Geometry: final body of the model. Coordinates: model frame, mm. Face numbers are marked on the shaded views. A direction names the side the tool comes from. Coordinates: 2 decimals unless noted, no trailing zeros. Order: outer loops, then holes, each group sorted by start corner. A loop starts at its lowest first (then second) coordinate and runs counter-clockwise, first axis right, second up. Notation, with made-up numbers: (82, -17.5) -> (89, -17.5) arc R26 cw to (89, 7.5) -> close; hole circle Ø2 at (-18, 83). An arc over 180 degrees is marked (long way). Answer in a Markdown table with one row per item. Add a question column.
1) Section query A-A on y = 11.25. Return the cut outline in (x, z), then the cut area to 3 significant figures.
2) Contact query for flat-ended pins moving along their axis: P1, Ø1.2, axis at x = -45.5, y = 11, coming from the +Z side; P2, Ø1, axis at x = -40, y = 8, coming from the -Z side; P3, Ø2, axis at x = -40, z = 30, coming from the -Y side. Output: stop coordinate, or through.
3) Section query C-C on y = 0. Return the cut outline in (x, z), then the cut area to 3 significant figures.
4) Section query B-B on y = -2.75. Return the cut outline in (x, z), then the cut area to 3 significant figures.
5) Pull-direction query (Z, two-part tool) for the marked faces 1, 2 and 3; classes: +Z half, -Z half, draft (parallel to the pull), parting line (faces both ways), or undercut.
6) Ray query, line 1 (Z direction, x = -39, y = -3.25); line 2 (Z direction, x = -41.5, y = -2.5); line 3 (Z direction, x = -41.5, y = 17.5). Return the intervals inside material, ascending. Write a range as from..to.
7) Set-up query: the marked faces 4, 5, 6, 7 and 8. Return all of +Z, -Z, +X, -X, +Y, -Y with unobstructed straight access to the full face (end or side cutting, diameter ignored); none if empty.
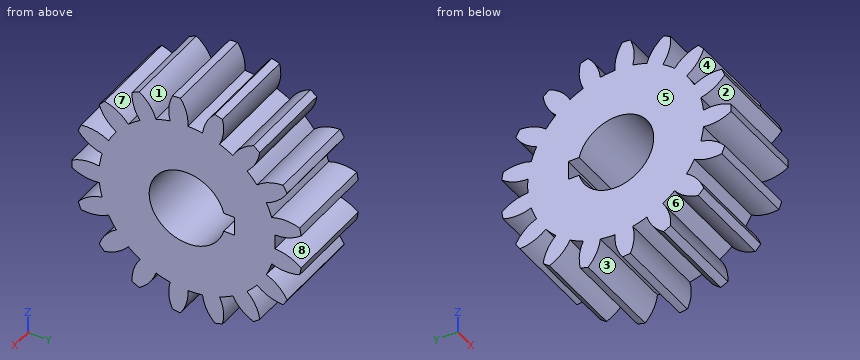
```python
from build123d import *

# Parameters (mm, degrees)
SPUR_START             = -48.138720077
SPUR_GEAR_AI_OUTLINE_R = 3.96875
SPUR_GEAR_AI_DEPTH     = 9.525
SKETCH1_W              = 2
SKETCH1_H              = 2
CUT_EXTRUDE1_DEPTH     = 39.960158194


# Read off the part's stored shape, not the designer's step: spur gear_ai
with BuildPart() as part:
    # spur gear_ai outline → spur gear_ai (new body)
    with BuildSketch(Plane.YZ.offset(SPUR_START)):
        with BuildLine():
            ThreePointArc((17.012312953, 13.95653765), (17.238554936, 14.308167954), (17.452476746, 14.667426586))
            ThreePointArc((17.452476746, 14.667426586), (16.531280061, 15.83450279), (15.268831698, 16.619929001))
            ThreePointArc((15.268831698, 16.619929001), (15.578265643, 17.328851589), (15.827189257, 18.061216004))
            ThreePointArc((15.827189257, 18.061216004), (17.289288072, 17.791147015), (18.756314792, 18.033020543))
            ThreePointArc((18.756314792, 18.033020543), (18.840255641, 18.442634067), (18.909952602, 18.854910235))
            ThreePointArc((18.909952602, 18.854910235), (17.629365722, 19.61040176), (16.168439009, 19.886740939))
            ThreePointArc((16.168439009, 19.886740939), (16.200885193, 20.659571999), (16.168439009, 21.43240306))
            ThreePointArc((16.168439009, 21.43240306), (17.629365722, 21.708742239), (18.909952602, 22.464233764))
            ThreePointArc((18.909952602, 22.464233764), (18.840255641, 22.876509932), (18.756314792, 23.286123456))
            ThreePointArc((18.756314792, 23.286123456), (17.289288072, 23.527996984), (15.827189257, 23.257927995))
            ThreePointArc((15.827189257, 23.257927995), (15.578265643, 23.99029241), (15.268831698, 24.699214998))
            ThreePointArc((15.268831698, 24.699214998), (16.531280061, 25.484641209), (17.452476746, 26.651717413))
            ThreePointArc((17.452476746, 26.651717413), (17.238554936, 27.010976045), (17.012312953, 27.362606349))
            ThreePointArc((17.012312953, 27.362606349), (15.55697648, 27.05819552), (14.291170111, 26.278192676))
            ThreePointArc((14.291170111, 26.278192676), (13.794495212, 26.871180574), (13.249864274, 27.420450766))
            ThreePointArc((13.249864274, 27.420450766), (14.143333641, 28.608887845), (14.580727415, 30.029928621))
            ThreePointArc((14.580727415, 30.029928621), (14.251472081, 30.287649847), (13.913484198, 30.533807309))
            ThreePointArc((13.913484198, 30.533807309), (12.666389228, 29.724224493), (11.767829468, 28.5396315))
            ThreePointArc((11.767829468, 28.5396315), (11.090481981, 28.913156579), (10.384209477, 29.228592392))
            ThreePointArc((10.384209477, 29.228592392), (10.788031858, 30.659535328), (10.682550269, 32.142621244))
            ThreePointArc((10.682550269, 32.142621244), (10.282429168, 32.263998384), (9.878342522, 32.371438077))
            ThreePointArc((9.878342522, 32.371438077), (9.00791614, 31.166021918), (8.597958464, 29.736824624))
            ThreePointArc((8.597958464, 29.736824624), (7.831417921, 29.840440252), (7.058889866, 29.879440332))
            ThreePointArc((7.058889866, 29.879440332), (6.918526812, 31.359632351), (6.284415731, 32.704464437))
            ThreePointArc((6.284415731, 32.704464437), (5.867467436, 32.673104837), (5.451856166, 32.627316432))
            ThreePointArc((5.451856166, 32.627316432), (5.075654279, 31.188865063), (5.209665743, 29.708084482))
            ThreePointArc((5.209665743, 29.708084482), (4.457457692, 29.527796795), (3.72300828, 29.285093965))
            ThreePointArc((3.72300828, 29.285093965), (3.057416599, 30.614626934), (1.980316242, 31.639578163))
            ThreePointArc((1.980316242, 31.639578163), (1.60285193, 31.45971711), (1.231846643, 31.266884587))
            ThreePointArc((1.231846643, 31.266884587), (1.4006774, 29.789668835), (2.060559012, 28.45729259))
            ThreePointArc((2.060559012, 28.45729259), (1.424273318, 28.017450439), (0.827094013, 27.52582306))
            ThreePointArc((0.827094013, 27.52582306), (-0.273834451, 28.525136184), (-1.648455712, 29.091781215))
            ThreePointArc((-1.648455712, 29.091781215), (-1.935457393, 28.78770994), (-2.211750379, 28.473876399))
            ThreePointArc((-2.211750379, 28.473876399), (-1.520688507, 27.157402438), (-0.424057414, 26.153375324))
            ThreePointArc((-0.424057414, 26.153375324), (-0.858486842, 25.513381828), (-1.237743667, 24.839226903))
            ThreePointArc((-1.237743667, 24.839226903), (-2.625322424, 25.373357406), (-4.111814371, 25.405167687))
            ThreePointArc((-4.111814371, 25.405167687), (-4.269592255, 25.017952702), (-4.41385804, 24.625503102))
            ThreePointArc((-4.41385804, 24.625503102), (-3.293896789, 23.647568035), (-1.908622321, 23.107489476))
            ThreePointArc((-1.908622321, 23.107489476), (-2.082523381, 22.353779304), (-2.19263699, 21.58814519))
            ThreePointArc((-2.19263699, 21.58814519), (-3.67946584, 21.58495579), (-5.077069498, 21.077635166))
            ThreePointArc((-5.077069498, 21.077635166), (-5.084314807, 20.659572), (-5.077069498, 20.241508833))
            ThreePointArc((-5.077069498, 20.241508833), (-3.67946584, 19.734188209), (-2.19263699, 19.730998809))
            ThreePointArc((-2.19263699, 19.730998809), (-2.082523381, 18.965364695), (-1.908622321, 18.211654523))
            ThreePointArc((-1.908622321, 18.211654523), (-3.293896789, 17.671575965), (-4.41385804, 16.693640897))
            ThreePointArc((-4.41385804, 16.693640897), (-4.269592255, 16.301191297), (-4.111814371, 15.913976312))
            ThreePointArc((-4.111814371, 15.913976312), (-2.625322424, 15.945786593), (-1.237743667, 16.479917096))
            ThreePointArc((-1.237743667, 16.479917096), (-0.858486842, 15.805762171), (-0.424057414, 15.165768676))
            ThreePointArc((-0.424057414, 15.165768676), (-1.520688507, 14.161741561), (-2.211750379, 12.8452676))
            ThreePointArc((-2.211750379, 12.8452676), (-1.935457393, 12.531434059), (-1.648455712, 12.227362784))
            ThreePointArc((-1.648455712, 12.227362784), (-0.273834451, 12.794007815), (0.827094013, 13.793320939))
            ThreePointArc((0.827094013, 13.793320939), (1.424273319, 13.301693561), (2.060559012, 12.861851409))
            ThreePointArc((2.060559012, 12.861851409), (1.4006774, 11.529475164), (1.231846643, 10.052259412))
            ThreePointArc((1.231846643, 10.052259412), (1.60285193, 9.859426889), (1.980316242, 9.679565836))
            ThreePointArc((1.980316242, 9.679565836), (3.057416599, 10.704517066), (3.72300828, 12.034050035))
            ThreePointArc((3.72300828, 12.034050035), (4.457457692, 11.791347204), (5.209665743, 11.611059517))
            ThreePointArc((5.209665743, 11.611059517), (5.075654279, 10.130278936), (5.451856166, 8.691827567))
            ThreePointArc((5.451856166, 8.691827567), (5.867467436, 8.646039163), (6.284415731, 8.614679562))
            ThreePointArc((6.284415731, 8.614679562), (6.918526812, 9.959511648), (7.058889866, 11.439703667))
            ThreePointArc((7.058889866, 11.439703667), (7.831417921, 11.478703747), (8.597958464, 11.582319375))
            ThreePointArc((8.597958464, 11.582319375), (9.00791614, 10.153122081), (9.878342522, 8.947705923))
            ThreePointArc((9.878342522, 8.947705923), (10.282429168, 9.055145615), (10.682550269, 9.176522755))
            ThreePointArc((10.682550269, 9.176522755), (10.788031858, 10.659608671), (10.384209477, 12.090551607))
            ThreePointArc((10.384209477, 12.090551607), (11.090481981, 12.405987421), (11.767829468, 12.779512499))
            ThreePointArc((11.767829468, 12.779512499), (12.666389228, 11.594919506), (13.913484198, 10.78533669))
            ThreePointArc((13.913484198, 10.78533669), (14.251472081, 11.031494152), (14.580727415, 11.289215378))
            ThreePointArc((14.580727415, 11.289215378), (14.143333641, 12.710256154), (13.249864274, 13.898693234))
            ThreePointArc((13.249864274, 13.898693234), (13.794495212, 14.447963426), (14.291170111, 15.040951324))
            ThreePointArc((14.291170111, 15.040951324), (15.55697648, 14.260948479), (17.012312953, 13.95653765))
        make_face()
        with Locations((6.980685193, 20.659572)):
            Circle(SPUR_GEAR_AI_OUTLINE_R, mode=Mode.SUBTRACT)
    extrude(amount=SPUR_GEAR_AI_DEPTH)

    # Sketch1 → Cut-Extrude1 (cut, through all)
    with BuildSketch(Plane(origin=(-38.613720077, 0, 0), x_dir=(0, 0, -1), z_dir=(1, 0, 0))):
        with Locations((-20.659572, 10.949435193)):
            Rectangle(SKETCH1_W, SKETCH1_H)
    extrude(amount=-CUT_EXTRUDE1_DEPTH, mode=Mode.SUBTRACT)


solid = part.part
```
Result:
| question | item | result |
|---|---|---|
| 1 | outline | (-48.14, 12.49) -> (-38.61, 12.49) -> (-38.61, 19.66) -> (-48.14, 19.66) -> close; (-48.14, 21.66) -> (-38.61, 21.66) -> (-38.61, 28.83) -> (-48.14, 28.83) -> close |
| 1 | area | 137 mm2 |
| 2 | P1 | z = 32.23 |
| 2 | P2 | z = 11.45 |
| 2 | P3 | y = -1.74 |
| 3 | outline | (-48.14, 12.98) -> (-38.61, 12.98) -> (-38.61, 28.34) -> (-48.14, 28.34) -> close |
| 3 | area | 146 mm2 |
| 4 | outline | (-48.14, 15.92) -> (-38.61, 15.92) -> (-38.61, 17.95) -> (-48.14, 17.95) -> close; (-48.14, 19.67) -> (-38.61, 19.67) -> (-38.61, 21.65) -> (-48.14, 21.65) -> close; (-48.14, 23.37) -> (-38.61, 23.37) -> (-38.61, 25.4) -> (-48.14, 25.4) -> close |
| 4 | area | 57.4 mm2 |
| 5 | face 1 | +Z half |
| 5 | face 2 | undercut |
| 5 | face 3 | -Z half |
| 6 | line 1 | 15.87..17.7, 19.68..21.64, 23.62..25.45 |
| 6 | line 2 | 15.97..18.05, 19.69..21.63, 23.27..25.35 |
| 6 | line 3 | 17.79..19.66, 21.66..23.52 |
| 7 | face 4 | +X, -X, -Y |
| 7 | face 5 | +Z, -Z, -X, +Y, -Y |
| 7 | face 6 | +X, -X |
| 7 | face 7 | +Z, +X, -X |
| 7 | face 8 | +X, -X, +Y |
